Source: CAD feature listing. Evaluate the final solid. Frame: model axes, mm. A direction names the side the tool comes from. Coordinates: 2 decimals unless noted, no trailing zeros. Order: outer loops, then holes, each group sorted by start corner. A loop starts at its lowest first (then second) coordinate and runs counter-clockwise, first axis right, second up.
```python
from build123d import *

# Parameters (mm, degrees)
PAD007_DEPTH = 0.8
PAD006_DEPTH = 1


with BuildPart() as obj1:
    # Sketch013 → Pad007 (new body)
    with BuildSketch(Plane.XY):
        Polygon((-14.5, 2.5), (-14.5, -2.5), (-10.5, -2.5), (-6, -6), (-6, 6), (-10.5, 2.5), align=None)
    extrude(amount=PAD007_DEPTH)


with BuildPart() as obj1_1:
    # Body008 placement: moved
    add(obj1.part.moved(Location((10.2, 0, 2))))


with BuildPart() as obj2:
    # Sketch014 → Pad006 (new body)
    with BuildSketch(Plane.XY):
        Polygon((-5.303301, 6.303301), (0, 1), (5.303301, 6.303301), (6.303301, 5.303301), (1, 0), (6.303301, -5.303301), (5.303301, -6.303301), (0, -1), (-5.303301, -6.303301), (-6.303301, -5.303301), (-1, 0), (-6.303301, 5.303301), align=None)
    extrude(amount=PAD006_DEPTH)


with BuildPart() as obj2_1:
    # Body009 placement: moved
    add(obj2.part.moved(Location((0, 0, 2))))

    # Fusion003: union obj1
    add(obj1_1.part)


solid = obj2_1.part
```
1. Pin query (flat end, axial travel): P1, Ø0.6, axis at x = -4, z = 2.5, coming from the -Y side; P2, Ø0.6, axis at x = -4, z = 2.5, coming from the +Y side. Return the tip coordinate at first contact, or that it passes through.
Findings:
P1: stops at y = -5.3
P2: stops at y = 5.3
2. Section query A-A on y = 4.25. Return loops of the section in (x, z), plus the area to 3 significant figures.
Findings:
outline: (-5.25, 2) - (-3.25, 2) - (-3.25, 3) - (-5.25, 3) - close; (1.95, 2) - (5.25, 2) - (5.25, 3) - (3.25, 3) - (3.25, 2.8) - (1.95, 2.8) - close
area: 5.04 mm2
3. Ray query, line 1 (Y direction, x = -4.25, z = 2.7); line 2 (X direction, y = 2, z = 2.25); line 3 (X direction, y = -3, z = 2.95). Return the intervals inside material, ascending.
Findings:
line 1: y = -5.25 to -3.25, -2.5 to 2.5, 3.25 to 5.25
line 2: x = -4.3 to 4.2
line 3: x = -4 to -2, 2 to 4
4. Section query B-B on x = 5. Return loops of the section in (y, z), plus the area to 3 significant figures.
Findings:
outline: (-6, 2) - (-4, 2) - (-4, 3) - (-6, 3) - close; (4, 2) - (6, 2) - (6, 3) - (4, 3) - close
area: 4.00 mm2
5. Access query for faces 5 (the face through (-3, 0, 2.8)), 6 (the face through (3, 0, 2.8)), 7 (the face through (1, 3, 2.8)). Directions: +Z, -Z, +X, -X, +Y, -Y. A direction counts if a zero-diameter tool reaches every point of the face in a straight line with its end or side. Return the directions, or none.
Findings:
face 5: +Z, -X
face 6: +Z, +X
face 7: +Z, +Y
6. Section query C-C on x = -0.75. Return loops of the section in (y, z).
Findings:
outline: (-2.5, 2) - (2.5, 2) - (2.5, 2.8) - (1.75, 2.8) - (1.75, 3) - (-1.75, 3) - (-1.75, 2.8) - (-2.5, 2.8) - close
7. Draft query along X for faces 1 (the face through (1.918, -4.226, 2.394)), 2 (the face through (0, 0, 3)), 3 (the face through (1, -3, 2.8)), 4 (the face through (4.8, -3.8, 2.6)). Return one class per face: released by +X, released by -X, zero draft, split by the parting line, or undercut.
Findings:
face 1: undercut
face 2: zero draft
face 3: undercut
face 4: released by +X
8. Section query D-D on z = 2.2. Return loops of the section in (x, y), plus the area to 3 significant figures.
Findings:
outline: (-6.3, -5.3) - (-5.3, -6.3) - (-1.5, -2.5) - (-0.3, -2.5) - (4.2, -6) - (4.2, -5.2) - (5.3, -6.3) - (6.3, -5.3) - (4.2, -3.2) - (4.2, 3.2) - (6.3, 5.3) - (5.3, 6.3) - (4.2, 5.2) - (4.2, 6) - (-0.3, 2.5) - (-1.5, 2.5) - (-5.3, 6.3) - (-6.3, 5.3) - (-3.5, 2.5) - (-4.3, 2.5) - (-4.3, -2.5) - (-3.5, -2.5) - close
area: 77.9 mm2
